```python
from build123d import *

# Parameters (mm, degrees)
SKETCH1_R           = 3.5
BOSS_EXTRUDE1_DEPTH = 23
BOSS_EXTRUDE2_START = 16
SKETCH1_3_W         = 4.65
SKETCH1_3_H         = 12.5
BOSS_EXTRUDE2_DEPTH = 3
BOSS_EXTRUDE3_START = 23
SKETCH1_4_R         = 6.25
BOSS_EXTRUDE3_DEPTH = 4
BOSS_EXTRUDE4_START = 27
SKETCH1_5_R         = 3.5
BOSS_EXTRUDE4_DEPTH = 5.6


with BuildPart() as part:
    # Sketch1 → Boss-Extrude1 (new body)
    # profile 1 of 8: a face of its own
    with BuildSketch(Plane(origin=(0, 0, 0), x_dir=(1, 0, 0), z_dir=(0, 1, 0))):
        with BuildLine():
            Line((-4.490881441, 6.284153005), (-10.740881441, 6.284153005))
            Line((-10.740881441, 6.284153005), (-10.740881441, 0.034153005))
            ThreePointArc((-10.740881441, 0.034153005), (-8.910298823, 4.453570388), (-4.490881441, 6.284153005))
        make_face()
    # profile 2 of 8: a face of its own
    with BuildSketch(Plane(origin=(0, 0, 0), x_dir=(1, 0, 0), z_dir=(0, 1, 0))):
        with BuildLine():
            ThreePointArc((0.759118559, 3.425317997), (-1.501925201, 5.523109245), (-4.490881441, 6.284153005))
            ThreePointArc((-4.490881441, 6.284153005), (-8.910298823, 4.453570388), (-10.740881441, 0.034153005))
            ThreePointArc((-10.740881441, 0.034153005), (-8.910298823, -4.385264377), (-4.490881441, -6.215846995))
            ThreePointArc((-4.490881441, -6.215846995), (-1.501925201, -5.454803234), (0.759118559, -3.357011986))
            Line((0.759118559, -3.357011986), (0.759118559, 3.425317997))
        make_face()
        with Locations((-4.490881441, 0.034153005)):
            Circle(SKETCH1_R, mode=Mode.SUBTRACT)
    # profile 3 of 8: a face of its own
    with BuildSketch(Plane(origin=(0, 0, 0), x_dir=(1, 0, 0), z_dir=(0, 1, 0))):
        with BuildLine():
            Line((12.259118559, 6.284153005), (0.759118559, 6.284153005))
            Line((0.759118559, 6.284153005), (0.759118559, 3.425317997))
            ThreePointArc((0.759118559, 3.425317997), (1.503907964, 1.801919958), (1.759118559, 0.034153005))
            ThreePointArc((1.759118559, 0.034153005), (1.503907964, -1.733613948), (0.759118559, -3.357011986))
            Line((0.759118559, -3.357011986), (0.759118559, -6.215846995))
            Line((0.759118559, -6.215846995), (12.259118559, -6.215846995))
            Line((12.259118559, -6.215846995), (12.259118559, 6.284153005))
        make_face()
    # profile 4 of 8: a face of its own
    with BuildSketch(Plane(origin=(0, 0, 0), x_dir=(1, 0, 0), z_dir=(0, 1, 0))):
        with BuildLine():
            ThreePointArc((0.759118559, -3.357011986), (-1.501925201, -5.454803234), (-4.490881441, -6.215846995))
            Line((-4.490881441, -6.215846995), (0.759118559, -6.215846995))
            Line((0.759118559, -6.215846995), (0.759118559, -3.357011986))
        make_face()
    # profile 5 of 8: a face of its own
    with BuildSketch(Plane(origin=(0, 0, 0), x_dir=(1, 0, 0), z_dir=(0, 1, 0))):
        with BuildLine():
            Line((0.759118559, 6.284153005), (-4.490881441, 6.284153005))
            ThreePointArc((-4.490881441, 6.284153005), (-1.501925201, 5.523109245), (0.759118559, 3.425317997))
            Line((0.759118559, 3.425317997), (0.759118559, 6.284153005))
        make_face()
    # profile 6 of 8: a face of its own
    with BuildSketch(Plane(origin=(0, 0, 0), x_dir=(1, 0, 0), z_dir=(0, 1, 0))):
        with BuildLine():
            ThreePointArc((1.759118559, 0.034153005), (1.503907964, 1.801919958), (0.759118559, 3.425317997))
            Line((0.759118559, 3.425317997), (0.759118559, -3.357011986))
            ThreePointArc((0.759118559, -3.357011986), (1.503907964, -1.733613948), (1.759118559, 0.034153005))
        make_face()
    # profile 7 of 8: a face of its own
    with BuildSketch(Plane(origin=(0, 0, 0), x_dir=(1, 0, 0), z_dir=(0, 1, 0))):
        with Locations((-4.490881441, 0.034153005)):
            Circle(SKETCH1_R)
    # profile 8 of 8: a face of its own
    with BuildSketch(Plane(origin=(0, 0, 0), x_dir=(1, 0, 0), z_dir=(0, 1, 0))):
        with BuildLine():
            ThreePointArc((-4.490881441, -6.215846995), (-8.910298823, -4.385264377), (-10.740881441, 0.034153005))
            Line((-10.740881441, 0.034153005), (-10.740881441, -6.215846995))
            Line((-10.740881441, -6.215846995), (-4.490881441, -6.215846995))
        make_face()
    extrude(amount=BOSS_EXTRUDE1_DEPTH)

    # Sketch1<3> → Boss-Extrude2 (add)
    with BuildSketch(Plane(origin=(0, 0, 0), x_dir=(1, 0, 0), z_dir=(0, 1, 0)).offset(BOSS_EXTRUDE2_START)):
        with Locations((-13.065881441, 0.034153005)):
            Rectangle(SKETCH1_3_W, SKETCH1_3_H)
        with Locations((14.584118559, 0.034153005)):
            Rectangle(SKETCH1_3_W, SKETCH1_3_H)
    extrude(amount=BOSS_EXTRUDE2_DEPTH)

    # Sketch1<4> → Boss-Extrude3 (add)
    with BuildSketch(Plane(origin=(0, 0, 0), x_dir=(1, 0, 0), z_dir=(0, 1, 0)).offset(BOSS_EXTRUDE3_START)):
        with Locations(Location((-4.490881441, 0.034153005, 0), (0, 0, 270))):
            Circle(SKETCH1_4_R)
    extrude(amount=BOSS_EXTRUDE3_DEPTH)

    # Sketch1<5> → Boss-Extrude4 (add)
    with BuildSketch(Plane(origin=(0, 0, 0), x_dir=(1, 0, 0), z_dir=(0, 1, 0)).offset(BOSS_EXTRUDE4_START)):
        with Locations(Location((-4.490881441, 0.034153005, 0), (0, 0, 270))):
            Circle(SKETCH1_5_R)
    extrude(amount=BOSS_EXTRUDE4_DEPTH)


solid = part.part
```
For this review, take the finished solid that the model builds, in its own axes (mm). A direction names the side the tool comes from. Round coordinates to 2 decimals unless told otherwise and drop trailing zeros. Write each loop counter-clockwise with the first axis right and the second up, starting at its lowest first coordinate (ties: lowest second). Pieces come first, ordered by that corner, then holes. Notation, with made-up numbers: M 84.5,-1 L 110.5,-1 A18 cw 110.5,12 Z; hole C 68,54 d11. An arc over 180 degrees is marked long. One line per item, written item: value. Start each with the question number.
(1) Insertion check: pin 1 (6 mm diameter, centred on y = 15, z = -4.5, fed in from -X); pin 2 (2 mm diameter, centred on y = 7, z = -1.5, fed in from +X); pin 3 (1.2 mm diameter, centred on y = 21, z = -3, fed in from -X); pin 4 (1.4 mm diameter, centred on x = -13, z = -1.5, fed in from -Y). Each pin has a flat end and moves straight along its axis. Give the tip position at first contact, or say it passes through.
(2) Machinability: for faces 1 (the flat face through (12.259, 8, 0)), 2 (the flat face through (12.259, 21, 0)), 3 (the flat face through (-10.741, 8, 0)), 4 (the flat face through (-10.741, 21, 0)), 5 (the cylindrical face through (-7.596, 29.761, 1.581)), which of the approach directions +Z, -Z, +X, -X, +Y, -Y give a long, thin tool a straight path to every point of the face, cutting with its end or side? Answer none if there is none.
(3) We need section C-C (y = 29.5). Give the boundary of the cut face in (x, z), and give its area (3 significant figures).
(4) We need section B-B (x = 3). Give the boundary of the cut face in (y, z).
(5) We need section A-A (z = -4). Give the boundary of the cut face in (x, y), and give its area (3 significant figures).
(6) Wall thickness on line 1 (X direction, y = 4.5, z = 0.5); line 2 (Y direction, x = -2, z = -3.25); line 3 (Y direction, x = 8.5, z = -5.25): over which ranges is each line inside the solid? List them lowest first.
(7) We need section D-D (z = 1.5). Give the boundary of the cut face in (x, y), and give its area (3 significant figures).
Result:
1. pin 1: x = -15.39
1. pin 2: x = 12.26
1. pin 3: x = -10.74
1. pin 4: y = 16
2. face 1: +Z, -Z, +X, -Y
2. face 2: +Z, -Z, +X, +Y
2. face 3: +Z, -Z, -X, -Y
2. face 4: +Z, -Z, -X, +Y
2. face 5: +Y
3. outline: C -4.49,-0.03 d7
3. area: 38.5 mm²
4. outline: M 0,-6.28 L 23,-6.28 L 23,6.22 L 0,6.22 Z
5. outline: M -15.39,16 L -10.74,16 L -10.74,0 L 12.26,0 L 12.26,16 L 16.91,16 L 16.91,19 L 12.26,19 L 12.26,23 L 0.34,23 L 0.34,27 L -9.32,27 L -9.32,23 L -10.74,23 L -10.74,19 L -15.39,19 Z
5. area: 596 mm²
6. line 1: -10.74 to 12.26
6. line 2: 0 to 27
6. line 3: 0 to 23
7. outline: M -15.39,16 L -10.74,16 L -10.74,0 L 12.26,0 L 12.26,16 L 16.91,16 L 16.91,19 L 12.26,19 L 12.26,23 L 1.57,23 L 1.57,27 L -1.35,27 L -1.35,32.6 L -7.64,32.6 L -7.64,27 L -10.55,27 L -10.55,23 L -10.74,23 L -10.74,19 L -15.39,19 Z
7. area: 641 mm²
